Read the model definition and answer for the solid it produces. Units are mm, in the model's axes. A direction names the side the tool comes from. Give positions to 0.01 mm unless a question says otherwise; leave off trailing zeros. Order: outer loops, then holes, each group sorted by start corner. A loop starts at its lowest first (then second) coordinate and runs counter-clockwise, first axis right, second up.
Item 1: Which of the six approach directions +Z, -Z, +X, -X, +Y, -Y give full straight-line access (tool end or side, diameter ignored) to faces 1 (the face through (6, 11, -0.25)), 2 (the face through (0, 12, 10)), 3 (the face through (-15, 24, -1)), 4 (the face through (-7.73, 3.94, 14.5)), 5 (the face through (0, 7.4, -4.5))?
Item 2: A cutting plane is placed at B-B (y = 14). Write down the section's boundary in (x, z), plus the area to 3 significant figures.
Item 3: The mould has two halves that part along Z. Classify faces 6 (the face through (-6, 11, -0.25)), 7 (the face through (23, 6, 21)), 8 (the face through (10, 22, -5)): +Z half, -Z half, draft (parallel to the pull), parting line (faces both ways), or undercut.
Item 4: A cutting plane is placed at A-A (x = 0). Write down the section's boundary in (y, z), plus the area to 4 significant figures.
Item 5: Find the intervals of material crossed by line 1 along Y through (x, z) = (-17, -8); line 2 along X through (y, z) = (6, 5); line 3 along X through (y, z) = (6, 17), in increasing order.
Item 6: A cutting plane is placed at D-D (z = 12). Write down the section's boundary in (x, y).
Item 7: Given pin 1 Ø3 at (x, z) = (4.5, -3) entering from +Y; pin 2 Ø11.5 at (x, y) = (17, 22) entering from +Z; pin 3 Ø8 at (x, y) = (-17, 22) entering from -Z; pin 4 Ø3 at (y, z) = (14.5, 8.5) entering from -X, each flat-ended and moving along its own axis, determine where each tip first touches the part or whether it passes through.
Item 8: A cutting plane is placed at C-C (y = 22). Write down the section's boundary in (x, z), plus the area to 3 significant figures.
from build123d import *

# Parameters (mm, degrees)
F0_W      = 48
F0_H      = 35
F0_R      = 10.5
F0_R_2    = 5
F0_R_3    = 2.5
F1_DEPTH  = 12
F2_DEPTH  = 8
F3_DEPTH  = 3
F5_DEPTH  = 3
F4_W      = 14
F4_H      = 15
F6_DEPTH  = 20
F7_R      = 2.5
F8_DEPTH  = 35.001
F9_R      = 5
F7_R_2    = 5
F10_DEPTH = 11


with BuildPart() as f1:
    # F0 (on Front) → F1 (new body)
    with BuildSketch(Plane.XZ):
        with Locations((0, 5.5)):
            Rectangle(F0_W, F0_H)
        Circle(F0_R, mode=Mode.SUBTRACT)
        with Locations((-12.5, 13)):
            Circle(F0_R_2, mode=Mode.SUBTRACT)
        with Locations((12.5, 13)):
            Circle(F0_R_2, mode=Mode.SUBTRACT)
        with Locations((-12.5, 13)):
            Circle(F0_R_2)
        with Locations((-12.5, 13)):
            Circle(F0_R_3, mode=Mode.SUBTRACT)
        with Locations((12.5, 13)):
            Circle(F0_R_2)
        with Locations((12.5, 13)):
            Circle(F0_R_3, mode=Mode.SUBTRACT)
        Circle(F0_R)
        with BuildLine():
            ThreePointArc((2.729107717, -3.5779842186), (-0.0063032395, -4.4999955855), (-2.7391205053, -3.5703247551))
            Line((-2.7391205053, -3.5703247551), (-4.5, -4.5869690054))
            ThreePointArc((-4.5, -4.5869690054), (-7.1256799724, -4.1571622293), (-6.2921852092, -1.6304616808))
            Line((-6.2921852092, -1.6304616808), (-4.5, -0.5957430678))
            Line((-4.5, -0.5957430678), (-4.5, 0))
            ThreePointArc((-4.5, 0), (-3.7417203652, 2.49990574), (-1.722431685, 4.1573103192))
            Line((-1.722431685, 4.1573103192), (-1.722431685, 6.1905988197))
            ThreePointArc((-1.722431685, 6.1905988197), (-0.1553134752, 8.2430942959), (1.75, 6.5))
            ThreePointArc((1.75, 6.5), (1.7460133012, 6.3819425903), (1.7340713692, 6.2644230769))
            Line((1.7340713692, 6.2644230769), (1.7340713692, 4.1524687219))
            ThreePointArc((1.7340713692, 4.1524687219), (3.9002621137, 2.2445390272), (4.4615521904, -0.5869855641))
            Line((4.4615521904, -0.5869855641), (6.222431685, -1.6036298143))
            ThreePointArc((6.222431685, -1.6036298143), (7.0610723284, -2.243947437), (7.3791651246, -3.25))
            ThreePointArc((7.3791651246, -3.25), (6.3999310593, -4.8211205791), (4.5581138401, -4.6339613961))
            Line((4.5581138401, -4.6339613961), (2.729107717, -3.5779842186))
        make_face(mode=Mode.SUBTRACT)
    extrude(amount=-F1_DEPTH)

    # F0 (on Front) → F2 (cut)
    with BuildSketch(Plane.XZ):
        with Locations((12.5, 13)):
            Circle(F0_R_2)
        with Locations((12.5, 13)):
            Circle(F0_R_3, mode=Mode.SUBTRACT)
        with Locations((-12.5, 13)):
            Circle(F0_R_2)
        with Locations((-12.5, 13)):
            Circle(F0_R_3, mode=Mode.SUBTRACT)
    extrude(amount=-F2_DEPTH, mode=Mode.SUBTRACT)

    # F0 (on Front) → F3 (cut)
    with BuildSketch(Plane.XZ):
        Circle(F0_R)
        with BuildLine():
            ThreePointArc((2.729107717, -3.5779842186), (-0.0063032395, -4.4999955855), (-2.7391205053, -3.5703247551))
            Line((-2.7391205053, -3.5703247551), (-4.5, -4.5869690054))
            ThreePointArc((-4.5, -4.5869690054), (-7.1256799724, -4.1571622293), (-6.2921852092, -1.6304616808))
            Line((-6.2921852092, -1.6304616808), (-4.5, -0.5957430678))
            Line((-4.5, -0.5957430678), (-4.5, 0))
            ThreePointArc((-4.5, 0), (-3.7417203652, 2.49990574), (-1.722431685, 4.1573103192))
            Line((-1.722431685, 4.1573103192), (-1.722431685, 6.1905988197))
            ThreePointArc((-1.722431685, 6.1905988197), (-0.1553134752, 8.2430942959), (1.75, 6.5))
            ThreePointArc((1.75, 6.5), (1.7460133012, 6.3819425903), (1.7340713692, 6.2644230769))
            Line((1.7340713692, 6.2644230769), (1.7340713692, 4.1524687219))
            ThreePointArc((1.7340713692, 4.1524687219), (3.9002621137, 2.2445390272), (4.4615521904, -0.5869855641))
            Line((4.4615521904, -0.5869855641), (6.222431685, -1.6036298143))
            ThreePointArc((6.222431685, -1.6036298143), (7.0610723284, -2.243947437), (7.3791651246, -3.25))
            ThreePointArc((7.3791651246, -3.25), (6.3999310593, -4.8211205791), (4.5581138401, -4.6339613961))
            Line((4.5581138401, -4.6339613961), (2.729107717, -3.5779842186))
        make_face(mode=Mode.SUBTRACT)
    extrude(amount=-F3_DEPTH, mode=Mode.SUBTRACT)

    # F4 (on face) → F5 (cut)
    with BuildSketch(Plane(origin=(0, 12, 0), x_dir=(-1, 0, 0), z_dir=(0, 1, 0))):
        with BuildLine():
            ThreePointArc((-4.4615521904, -0.5869855641), (-4.4804704843, -0.4187890156), (-4.4930501889, -0.25))
            Line((-4.4930501889, -0.25), (-7.3612159322, -0.25))
            Line((-7.3612159322, -0.25), (-9.0932667397, -3.25))
            Line((-9.0932667397, -3.25), (-7.3612159322, -6.25))
            Line((-7.3612159322, -6.25), (-3.897114317, -6.25))
            Line((-3.897114317, -6.25), (-2.4630314454, -3.7660956041))
            ThreePointArc((-2.4630314454, -3.7660956041), (-2.597772843, -3.6744491092), (-2.729107717, -3.5779842186))
            Line((-2.729107717, -3.5779842186), (-4.5581138401, -4.6339613961))
            ThreePointArc((-4.5581138401, -4.6339613961), (-7.1630480845, -4.0924387607), (-6.222431685, -1.6036298143))
            Line((-6.222431685, -1.6036298143), (-4.4615521904, -0.5869855641))
        make_face()
        with BuildLine():
            Line((1.7320508076, 9.5), (-1.7320508076, 9.5))
            Line((-1.7320508076, 9.5), (-3.4641016151, 6.5))
            Line((-3.4641016151, 6.5), (-2.0300187435, 4.0160956041))
            ThreePointArc((-2.0300187435, 4.0160956041), (-1.883279852, 4.0869618299), (-1.7340713692, 4.1524687219))
            Line((-1.7340713692, 4.1524687219), (-1.7340713692, 6.2644230769))
            ThreePointArc((-1.7340713692, 6.2644230769), (0.0373681121, 8.24960099), (1.722431685, 6.1905988197))
            Line((1.722431685, 6.1905988197), (1.722431685, 4.1573103192))
            ThreePointArc((1.722431685, 4.1573103192), (1.8775533158, 4.0895957681), (2.0300187435, 4.0160956041))
            Line((2.0300187435, 4.0160956041), (3.4641016151, 6.5))
            Line((3.4641016151, 6.5), (1.7320508076, 9.5))
        make_face()
        with BuildLine():
            Line((7.3612159322, -0.25), (4.5, -0.25))
            Line((4.5, -0.25), (4.5, -0.5957430678))
            Line((4.5, -0.5957430678), (6.2921852092, -1.6304616808))
            ThreePointArc((6.2921852092, -1.6304616808), (7.1256799724, -4.1571622293), (4.5, -4.5869690054))
            Line((4.5, -4.5869690054), (2.7391205053, -3.5703247551))
            ThreePointArc((2.7391205053, -3.5703247551), (2.6029171685, -3.6708067525), (2.4630314454, -3.7660956041))
            Line((2.4630314454, -3.7660956041), (3.897114317, -6.25))
            Line((3.897114317, -6.25), (7.3612159322, -6.25))
            Line((7.3612159322, -6.25), (9.0932667397, -3.25))
            Line((9.0932667397, -3.25), (7.3612159322, -0.25))
        make_face()
    extrude(amount=-F5_DEPTH, mode=Mode.SUBTRACT)

    # F4 (on face) → F6 (join)
    with BuildSketch(Plane(origin=(0, 12, 0), x_dir=(-1, 0, 0), z_dir=(0, 1, 0))):
        with Locations((-17, -4.5)):
            Rectangle(F4_W, F4_H)
        with Locations((17, -4.5)):
            Rectangle(F4_W, F4_H)
    extrude(amount=F6_DEPTH)

    # F7 (on face) → F8 (cut, through all)
    with BuildSketch(Plane(origin=(0, 0, -12), x_dir=(1, 0, 0), z_dir=(0, 0, -1))):
        with Locations((-17, -22)):
            Circle(F7_R)
        with Locations((17, -22)):
            Circle(F7_R)
    extrude(amount=-F8_DEPTH, mode=Mode.SUBTRACT)

    # F9
    f9_edges = [f1.edges().sort_by_distance(p)[0] for p in [
        (-24, 6, 23),
        (24, 6, 23),
    ]]
    fillet(f9_edges, radius=F9_R)

    # F7 (on face) → F10 (cut)
    with BuildSketch(Plane(origin=(0, 0, -12), x_dir=(1, 0, 0), z_dir=(0, 0, -1))):
        with Locations((-17, -22)):
            Circle(F7_R_2)
        with Locations((-17, -22)):
            Circle(F7_R, mode=Mode.SUBTRACT)
        with Locations((17, -22)):
            Circle(F7_R_2)
        with Locations((17, -22)):
            Circle(F7_R, mode=Mode.SUBTRACT)
    extrude(amount=-F10_DEPTH, mode=Mode.SUBTRACT)


solid = f1.part
Response values:
1. face 1: +Y
1. face 2: +Z, +Y
1. face 3: -Z
1. face 4: -Y
1. face 5: +Y, -Y
2. outline: (-24, -12) - (-10, -12) - (-10, 3) - (-24, 3) - close; (10, -12) - (24, -12) - (24, 3) - (10, 3) - close
2. area: 420 mm2
3. face 6: undercut
3. face 7: +Z half
3. face 8: draft
4. outline: (0, -12) - (12, -12) - (12, -4.5) - (3, -4.5) - (3, -10.5) - (0, -10.5) - close; (0, 10.5) - (3, 10.5) - (3, 8.25) - (9, 8.25) - (9, 9.5) - (12, 9.5) - (12, 23) - (0, 23) - close
4. area: 238.5 mm2
5. line 1: y = 0 to 17, 27 to 32
5. line 2: x = -24 to -1.72, 1.73 to 24
5. line 3: x = -24 to -15.5, -9.5 to 9.5, 15.5 to 24
6. outline: (-24, 0) - (-17.4, 0) - (-17.4, 8) - (-14.79, 8) - (-14.79, 12) - (-24, 12) - close; (-10.21, 8) - (-7.6, 8) - (-7.6, 0) - (7.6, 0) - (7.6, 8) - (10.21, 8) - (10.21, 12) - (-10.21, 12) - close; (14.79, 8) - (17.4, 8) - (17.4, 0) - (24, 0) - (24, 12) - (14.79, 12) - close
7. pin 1: stops at y = 9
7. pin 2: stops at z = 3
7. pin 3: stops at z = -1
7. pin 4: passes through
8. outline: (-24, -12) - (-22, -12) - (-22, -1) - (-19.5, -1) - (-19.5, 3) - (-24, 3) - close; (-14.5, -1) - (-12, -1) - (-12, -12) - (-10, -12) - (-10, 3) - (-14.5, 3) - close; (10, -12) - (12, -12) - (12, -1) - (14.5, -1) - (14.5, 3) - (10, 3) - close; (19.5, -1) - (22, -1) - (22, -12) - (24, -12) - (24, 3) - (19.5, 3) - close
8. area: 160 mm2
